```python
from build123d import *

# Parameters (mm, degrees)
F1_DEPTH = 5.25
F2_DEPTH = 4
F0_W     = 23.5
F0_H     = 4
F3_DEPTH = 2
F4_R     = 0.5
F5_R     = 2


with BuildPart() as f1:
    # F0 (on Front) → F1 (new body, symmetric)
    with BuildSketch(Plane.XZ):
        Polygon((-11.75, 0), (-15.5, 0), (-15.5, -5), (15.5, -5), (15.5, 0), (11.75, 0), align=None)
    extrude(amount=F1_DEPTH, both=True)



with BuildPart() as f2:
    # F0 (on Front) → F2 (new body, symmetric)
    with BuildSketch(Plane.XZ):
        Polygon((-14.5, 4), (-11.75, 4), (11.75, 4), (14.5, 4), (14.5, 5), (11.75, 5), (-11.75, 5), (-14.5, 5), align=None)
        Polygon((-14.5, 9), (-11.75, 9), (11.75, 9), (14.5, 9), (14.5, 10), (11.75, 10), (-11.75, 10), (-14.5, 10), align=None)
        Polygon((-14.5, 14), (-11.75, 14), (11.75, 14), (14.5, 14), (14.5, 15), (-14.5, 15), align=None)
    extrude(amount=F2_DEPTH, both=True)


with BuildPart() as f1_1:
    add(f1.part)

    add(f2.part)  # F3 merges F2
    # F0 (on Front) → F3 (join, symmetric)
    with BuildSketch(Plane.XZ):
        with Locations((0, 2)):
            Rectangle(F0_W, F0_H)
        with Locations((0, 7)):
            Rectangle(F0_W, F0_H)
        with Locations((0, 12)):
            Rectangle(F0_W, F0_H)
    extrude(amount=F3_DEPTH, both=True)

    # F4
    f4_edges = [f1_1.edges().sort_by_distance(p)[0] for p in [
        (15.5, -5.25, -2.5),
        (15.5, 5.25, -2.5),
        (-15.5, -5.25, -2.5),
        (-11.75, -2, 2),
        (-11.75, -2, 7),
        (-11.75, -2, 12),
        (11.75, -2, 2),
        (11.75, -2, 7),
        (11.75, -2, 12),
        (11.75, 2, 2),
        (11.75, 2, 7),
        (11.75, 2, 12),
        (-15.5, 5.25, -2.5),
        (-11.75, 2, 2),
        (-11.75, 2, 7),
        (-11.75, 2, 12),
    ]]
    fillet(f4_edges, radius=F4_R)

    # F5
    f5_edges = [f1_1.edges().sort_by_distance(p)[0] for p in [
        (-14.5, 4, 4.5),
        (-14.5, 4, 9.5),
        (-14.5, 4, 14.5),
        (-14.5, -4, 14.5),
        (-14.5, -4, 9.5),
        (-14.5, -4, 4.5),
        (14.5, -4, 14.5),
        (14.5, -4, 9.5),
        (14.5, -4, 4.5),
        (14.5, 4, 4.5),
        (14.5, 4, 9.5),
        (14.5, 4, 14.5),
    ]]
    fillet(f5_edges, radius=F5_R)


solid = f1_1.part
```
Check sheet for the modelled part. Datum: model origin and axes. Units: mm. A direction names the side the tool comes from. Round coordinates to 2 decimals unless told otherwise and drop trailing zeros. Loops run counter-clockwise (first coordinate to the right, second up) from the corner with the lowest first, then second, coordinate; pieces in that order, holes last. Notation, with made-up numbers: M 3,-39.75 L 52,-39.75 A16 ccw 52,-14.75 Z; hole C 39.25,76.25 d3. An arc over 180 degrees is marked long. Answer as a JSON object with one key per item and string values.
1. Mould release check, pull along Z, two halves, no side actions. Record for faces 1 (the flat face through (0, 3, 5)), 2 (the flat face through (-14.5, 0, 9.5)): pulls with the +Z half, pulls with the -Z half, needs draft (parallel to the pull), parting line crosses it, or undercut.
Reply:
{"face 1": "undercut", "face 2": "needs draft"}
2. Section check B-B (z = 11). Record the boundary of the cut face in (x, y), plus the area to 3 significant figures.
Reply:
{"outline": "M -11.75,-1.5 A0.5 ccw -11.25,-2 L 11.25,-2 A0.5 ccw 11.75,-1.5 L 11.75,1.5 A0.5 ccw 11.25,2 L -11.25,2 A0.5 ccw -11.75,1.5 Z", "area": "93.8 mm²"}
3. Access from +Z, -Z, +X, -X, +Y, -Y to the whole of each face (thin tool, end or side, straight path). Record for faces 3 (the flat face through (14.5, 0, 14.5)), 4 (the cylindrical face through (13.9, 3.43, 9.51)), 5 (the flat face through (-0.2, 4, 9.5)).
Reply:
{"face 3": "+Z, +X, +Y, -Y", "face 4": "+Z, +X, +Y", "face 5": "+Z, +X, -X, +Y"}
4. Section check C-C (x = -13). Record the boundary of the cut face in (y, z).
Reply:
{"outline": "M -5.25,-5 L 5.25,-5 L 5.25,0 L -5.25,0 Z; M -3.94,4 L 3.94,4 L 3.94,5 L -3.94,5 Z; M -3.94,9 L 3.94,9 L 3.94,10 L -3.94,10 Z; M -3.94,14 L 3.94,14 L 3.94,15 L -3.94,15 Z"}
5. Section check A-A (y = -0.5). Record the boundary of the cut face in (x, z).
Reply:
{"outline": "M -15.5,-5 L 15.5,-5 L 15.5,0 L 11.75,0 L 11.75,4 L 14.5,4 L 14.5,5 L 11.75,5 L 11.75,9 L 14.5,9 L 14.5,10 L 11.75,10 L 11.75,14 L 14.5,14 L 14.5,15 L -14.5,15 L -14.5,14 L -11.75,14 L -11.75,10 L -14.5,10 L -14.5,9 L -11.75,9 L -11.75,5 L -14.5,5 L -14.5,4 L -11.75,4 L -11.75,0 L -15.5,0 Z"}
6. Scan lines: line 1 (Z direction, x = 5, y = 3.5); line 2 (X direction, y = -1.25, z = 11); line 3 (Y direction, x = 7.5, z = 8.75). Record each from-to range of solid material in increasing order.
Reply:
{"line 1": "z = -5 to 0, 4 to 5, 9 to 10, 14 to 15", "line 2": "x = -11.75 to 11.75", "line 3": "y = -2 to 2"}
7. Section check D-D (x = -6). Record the boundary of the cut face in (y, z), plus the area to 4 significant figures.
Reply:
{"outline": "M -5.25,-5 L 5.25,-5 L 5.25,0 L 2,0 L 2,4 L 4,4 L 4,5 L 2,5 L 2,9 L 4,9 L 4,10 L 2,10 L 2,14 L 4,14 L 4,15 L -4,15 L -4,14 L -2,14 L -2,10 L -4,10 L -4,9 L -2,9 L -2,5 L -4,5 L -4,4 L -2,4 L -2,0 L -5.25,0 Z", "area": "124.5 mm²"}
8. Gauge pin test, flat ends, axial feed: P1, Ø1.5, axis at y = 3, z = 8.5, coming from the +X side; P2, Ø0.8, axis at y = -0.5, z = 9.5, coming from the -X side; P3, Ø1, axis at x = -2, z = 2.5, coming from the -Y side. Record the tip position at first contact, or that the pin passes through.
Reply:
{"P1": "stops at x = 14.45", "P2": "stops at x = -14.5", "P3": "stops at y = -2"}
